```python
from build123d import *

# Parameters (mm, degrees)
SKETCH1_W           = 660
SKETCH1_H           = 80
BOSS_EXTRUDE1_DEPTH = 6
SKETCH2_W           = 12.04
SKETCH2_H           = 26
CUT_EXTRUDE1_DEPTH  = 333.469547478
SKETCH3_W           = 6.04
SKETCH3_H           = 40
CUT_EXTRUDE2_DEPTH  = 333.469547478
SKETCH4_W           = 6.04
SKETCH4_H           = 40
CUT_EXTRUDE3_DEPTH  = 333.469547478


with BuildPart() as part:
    # Sketch1 → Boss-Extrude1 (new body)
    with BuildSketch(Plane.XY):
        Rectangle(SKETCH1_W, SKETCH1_H)
    extrude(amount=BOSS_EXTRUDE1_DEPTH)

    # Sketch2 → Cut-Extrude1 (cut, through all)
    with BuildSketch(Plane.XY.offset(6)):
        with Locations((-293.98, 27)):
            Rectangle(SKETCH2_W, SKETCH2_H)
        with Locations((-65.94, 27)):
            Rectangle(SKETCH2_W, SKETCH2_H)
        with Locations((66.1, 27)):
            Rectangle(SKETCH2_W, SKETCH2_H)
        with Locations((294.14, 27)):
            Rectangle(SKETCH2_W, SKETCH2_H)
    extrude(amount=-CUT_EXTRUDE1_DEPTH, mode=Mode.SUBTRACT)

    # Sketch3 → Cut-Extrude2 (cut, through all)
    with BuildSketch(Plane.XY.offset(6)):
        with Locations((-26.02, -20)):
            Rectangle(SKETCH3_W, SKETCH3_H)
        with Locations((26.02, -20)):
            Rectangle(SKETCH3_W, SKETCH3_H)
    extrude(amount=-CUT_EXTRUDE2_DEPTH, mode=Mode.SUBTRACT)

    # Sketch4 → Cut-Extrude3 (cut, through all)
    with BuildSketch(Plane.XY.offset(6)):
        with Locations((-189.94, -20)):
            Rectangle(SKETCH4_W, SKETCH4_H)
        with Locations((190.1, -20)):
            Rectangle(SKETCH4_W, SKETCH4_H)
    extrude(amount=-CUT_EXTRUDE3_DEPTH, mode=Mode.SUBTRACT)


solid = part.part
```
Source: CAD feature listing. Evaluate the final solid. Frame: model axes, mm. Coordinates: 2 decimals unless noted, no trailing zeros. Write each loop counter-clockwise with the first axis right and the second up, starting at its lowest first coordinate (ties: lowest second). Pieces come first, ordered by that corner, then holes. Notation, with made-up numbers: (67.5, -7.75) -> (120.5, -7.75) arc R26 ccw to (120.5, 29.25) -> close; hole circle Ø10 at (25, 14.25). An arc over 180 degrees is marked (long way). Return JSON: item names as keys, results as strings. Group by question number.
1) Section query B-B, the plane y = 26.5. Return loops of the section in (x, z), plus the area to 3 significant figures.
2) Ray query, line 1 along X through (y, z) = (-36, 3.8); line 2 along X through (y, z) = (19, 4.4). Return the intervals inside material, ascending.
3) Contact query for flat-ended pins moving along their axis: P1, Ø1.8, axis at x = -66, z = 4, coming from the +Y side; P2, Ø12, axis at x = 195, y = -3.5, coming from the -Z side; P3, Ø1.8, axis at x = 191.5, z = 4.5, coming from the -Y side. Output: stop coordinate, or through.
4) Section query A-A, the plane y = -33.5. Return loops of the section in (x, z), plus the area to 3 significant figures.
From the geometry:
{
 "1": {"outline": "(-330, 0) -> (-300, 0) -> (-300, 6) -> (-330, 6) -> close; (-287.96, 0) -> (-71.96, 0) -> (-71.96, 6) -> (-287.96, 6) -> close; (-59.92, 0) -> (60.08, 0) -> (60.08, 6) -> (-59.92, 6) -> close; (72.12, 0) -> (288.12, 0) -> (288.12, 6) -> (72.12, 6) -> close; (300.16, 0) -> (330, 0) -> (330, 6) -> (300.16, 6) -> close", "area": "3,670 mm²"},
 "2": {"line 1": "-330 to -192.96, -186.92 to -29.04, -23 to 23, 29.04 to 187.08, 193.12 to 330", "line 2": "-330 to -300, -287.96 to -71.96, -59.92 to 60.08, 72.12 to 288.12, 300.16 to 330"},
 "3": {"P1": "y = 14", "P2": "z = 0", "P3": "y = 0"},
 "4": {"outline": "(-330, 0) -> (-192.96, 0) -> (-192.96, 6) -> (-330, 6) -> close; (-186.92, 0) -> (-29.04, 0) -> (-29.04, 6) -> (-186.92, 6) -> close; (-23, 0) -> (23, 0) -> (23, 6) -> (-23, 6) -> close; (29.04, 0) -> (187.08, 0) -> (187.08, 6) -> (29.04, 6) -> close; (193.12, 0) -> (330, 0) -> (330, 6) -> (193.12, 6) -> close", "area": "3,820 mm²"}
}
